```python
from build123d import *

# Parameters (mm, degrees)
F2_R          = 30
F3_DEPTH      = 50.001
F3_DEPTH_BACK = 50.001
F4_R          = 30
F5_DEPTH      = 50.001
F5_DEPTH_BACK = 50.001
F6_R          = 30
F7_DEPTH      = 50.001
F7_DEPTH_BACK = 50.001


# Not quite as in the source:
# - a feature names something its author has since deleted; it is built from what else it names


with BuildPart() as f1:
    # F0 (on Front) → F1 (revolve)
    with BuildSketch(Plane.XZ):
        with BuildLine():
            Line((0, -50), (0, 0))
            Line((0, 0), (0, 50))
            ThreePointArc((0, 50), (-50, 0), (0, -50))
        make_face()
    revolve(axis=Axis((0, 0, 25), (0, 0, 1)))

    # F2 (on Front) → F3 (cut, two sides)
    with BuildSketch(Plane.XZ) as f3_sk:
        Circle(F2_R)
    extrude(amount=-F3_DEPTH, mode=Mode.SUBTRACT)
    extrude(f3_sk.sketch, amount=F3_DEPTH_BACK, mode=Mode.SUBTRACT)

    # F4 (on Right) → F5 (cut, two sides)
    with BuildSketch(Plane.YZ) as f5_sk:
        Circle(F4_R)
    extrude(amount=-F5_DEPTH, mode=Mode.SUBTRACT)
    extrude(f5_sk.sketch, amount=F5_DEPTH_BACK, mode=Mode.SUBTRACT)

    # F6 (on Top) → F7 (cut, two sides)
    with BuildSketch(Plane.XY) as f7_sk:
        Circle(F6_R)
    extrude(amount=F7_DEPTH, mode=Mode.SUBTRACT)
    extrude(f7_sk.sketch, amount=-F7_DEPTH_BACK, mode=Mode.SUBTRACT)

    # F8 (on Front) → F9 (revolve, cut)
    with BuildSketch(Plane.XZ):
        with BuildLine():
            Line((0, -45), (0, 0))
            Line((0, 0), (0, 45))
            ThreePointArc((0, 45), (-45, 0), (0, -45))
        make_face()
    revolve(axis=Axis((0, 0, 22.5), (0, 0, 1)), mode=Mode.SUBTRACT)


solid = f1.part
```
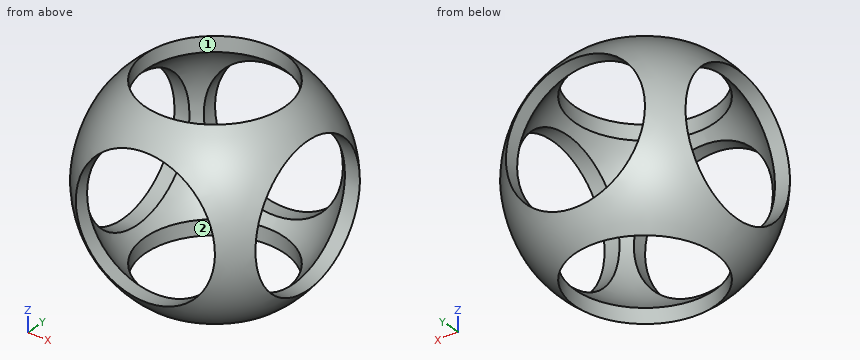
Here's how the part is built. I have some questions about the finished solid (model axes, mm). Face numbers are marked on the shaded views. Round coordinates to 2 decimals unless told otherwise and drop trailing zeros. Order: outer loops, then holes, each group sorted by start corner. A loop starts at its lowest first (then second) coordinate and runs counter-clockwise, first axis right, second up. Notation, with made-up numbers: (88, 89) -> (114, 89) arc R6 ccw to (114, 94) -> close; hole circle Ø3 at (71, 20). An arc over 180 degrees is marked (long way). Use a Markdown table: item, result. Add a question column.
(1) Suppose I cut it at D-D, the plane x = -32. Please give me the cut outline in (y, z).
(2) I need wall thicknesses on line 1 along Z through (x, y) = (-37, 0); line 2 along X through (y, z) = (-35, 0). Which ranges of each line are inside material? Lowest first, please.
(3) Suppose I cut it at C-C, the plane y = -31.5. Please give me the cut outline in (x, z).
(4) Suppose I cut it at A-A, the plane x = -18. Please give me the cut outline in (y, z), and give its area (3 significant figures).
(5) If we mould it in two halves opening along Y, with no side actions, what happens to the marked faces 1 and 2? For each: released by +Y, released by -Y, zero draft, split by the parting line, or undercut.
(6) Suppose I cut it at B-B, the plane z = 0. Please give me the cut outline in (x, y).
(7) For pin 1 Ø6 at (y, z) = (-30.5, 14) entering from +X; pin 2 Ø1 at (x, z) = (-28.5, -27.5) entering from -Y, each with a flat end and sliding along its axis, tell me the tip position at first contact or that it passes through.
Verdict:
| question | item | result |
|---|---|---|
| 1 | outline | circle Ø76.84 at (0, 0); hole circle Ø63.28 at (0, 0) |
| 2 | line 1 | -33.63 to -30, 30 to 33.63 |
| 2 | line 2 | -35.71 to -30, 30 to 35.71 |
| 3 | outline | circle Ø77.66 at (0, 0); hole circle Ø64.27 at (0, 0) |
| 4 | outline | (-40, -24) arc R46.65 ccw to (-24, -40) -> (-24, -33.54) arc R41.24 cw to (-33.54, -24) -> close; (-40, 24) -> (-33.54, 24) arc R41.24 cw to (-24, 33.54) -> (-24, 40) arc R46.65 ccw to start; (24, -40) arc R46.65 ccw to (40, -24) -> (33.54, -24) arc R41.24 cw to (24, -33.54) -> close; (24, 33.54) arc R41.24 cw to (33.54, 24) -> (40, 24) arc R46.65 ccw to (24, 40) -> close |
| 4 | area | 394 mm2 |
| 5 | face 1 | undercut |
| 5 | face 2 | undercut |
| 6 | outline | (-40, -30) arc R50 ccw to (-30, -40) -> (-30, -33.54) arc R45 cw to (-33.54, -30) -> close; (-40, 30) -> (-33.54, 30) arc R45 cw to (-30, 33.54) -> (-30, 40) arc R50 ccw to start; (30, -40) arc R50 ccw to (40, -30) -> (33.54, -30) arc R45 cw to (30, -33.54) -> close; (30, 33.54) arc R45 cw to (33.54, 30) -> (40, 30) arc R50 ccw to (30, 40) -> close |
| 7 | pin 1 | x = 39.57 |
| 7 | pin 2 | y = -31.16 |
